Could you check a few things on this drawing? It's one solid part, dimensions in mm from its lowest x, y, z. A direction names the side the tool comes from. Round coordinates to 2 decimals unless told otherwise and drop trailing zeros. Write each loop counter-clockwise with the first axis right and the second up, starting at its lowest first coordinate (ties: lowest second). Pieces come first, ordered by that corner, then holes. Notation, with made-up numbers: M -1,-4.75 L 57,-4.75 A22 ccw 57,32.25 Z; hole C 13.25,56.25 d4. An arc over 180 degrees is marked long. One line per question, with ' | ' between items. Start each with the question number.
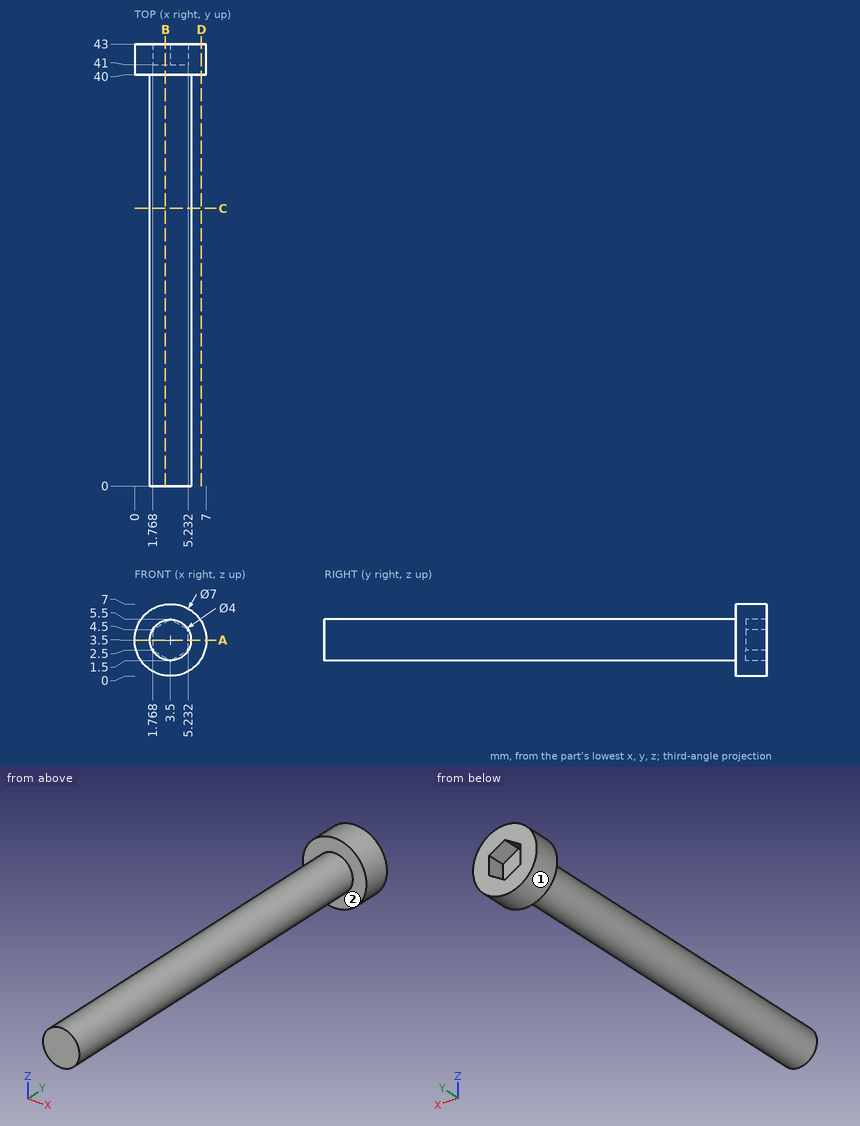
1. Suppose I cut it at B-B (x = 3). Write out the boundary of the cut face in (y, z).
2. I need wall thicknesses on line 1 along Y through (x, z) = (6.5, 3); line 2 along Y through (x, z) = (4.25, 3.75); line 3 along Z through (x, y) = (3.5, 29.5). Which ranges of each line are inside material? Lowest first, please. Write a range as from..to.
3. Suppose I cut it at A-A (z = 3.5). Write out the boundary of the cut face in (x, y), and give its area (3 significant figures).
4. Suppose I cut it at C-C (y = 27). Write out the boundary of the cut face in (x, z).
5. Suppose I cut it at D-D (x = 6.5). Write out the boundary of the cut face in (y, z).
6. I'm going to push a flat-ended pin straight in: P1, Ø3, axis at x = 4, z = 3.5, coming from the +Y side. Where does the tip first touch, or does it pass through?
7. Which directions (+Z, -Z, +X, -X, +Y, -Y) give clear straight access to the entire face, cutting with the end or side of a thin tool? Please do the marked faces 1 and 2.
Computed:
1) outline: M 0,1.56 L 40,1.56 L 40,0.04 L 43,0.04 L 43,1.79 L 41,1.79 L 41,5.21 L 43,5.21 L 43,6.96 L 40,6.96 L 40,5.44 L 0,5.44 Z
2) line 1: y = 40..43 | line 2: y = 0..41 | line 3: z = 1.5..5.5
3) outline: M 0,40 L 1.5,40 L 1.5,0 L 5.5,0 L 5.5,40 L 7,40 L 7,43 L 5.23,43 L 5.23,41 L 1.77,41 L 1.77,43 L 0,43 Z | area: 174 mm²
4) outline: C 3.5,3.5 d4
5) outline: M 40,1.7 L 43,1.7 L 43,5.3 L 40,5.3 Z
6) P1: stops at y = 43
7) face 1: +Y, -Y | face 2: -Y
